The figure shows three views and two pictorial views of one solid part (mm, origin at its lowest corner). Answer the questions. Give positions to 0.01 mm unless a question says otherwise; leave off trailing zeros. Write each loop counter-clockwise with the first axis right and the second up, starting at its lowest first coordinate (ties: lowest second). Pieces come first, ordered by that corner, then holes. Notation, with made-up numbers: (23.5, -0.5) -> (32.5, -0.5) arc R35 ccw to (32.5, 34.5) -> close; hole circle Ø1 at (86.5, 7). An arc over 180 degrees is marked (long way). Use a Markdown table: item, result.
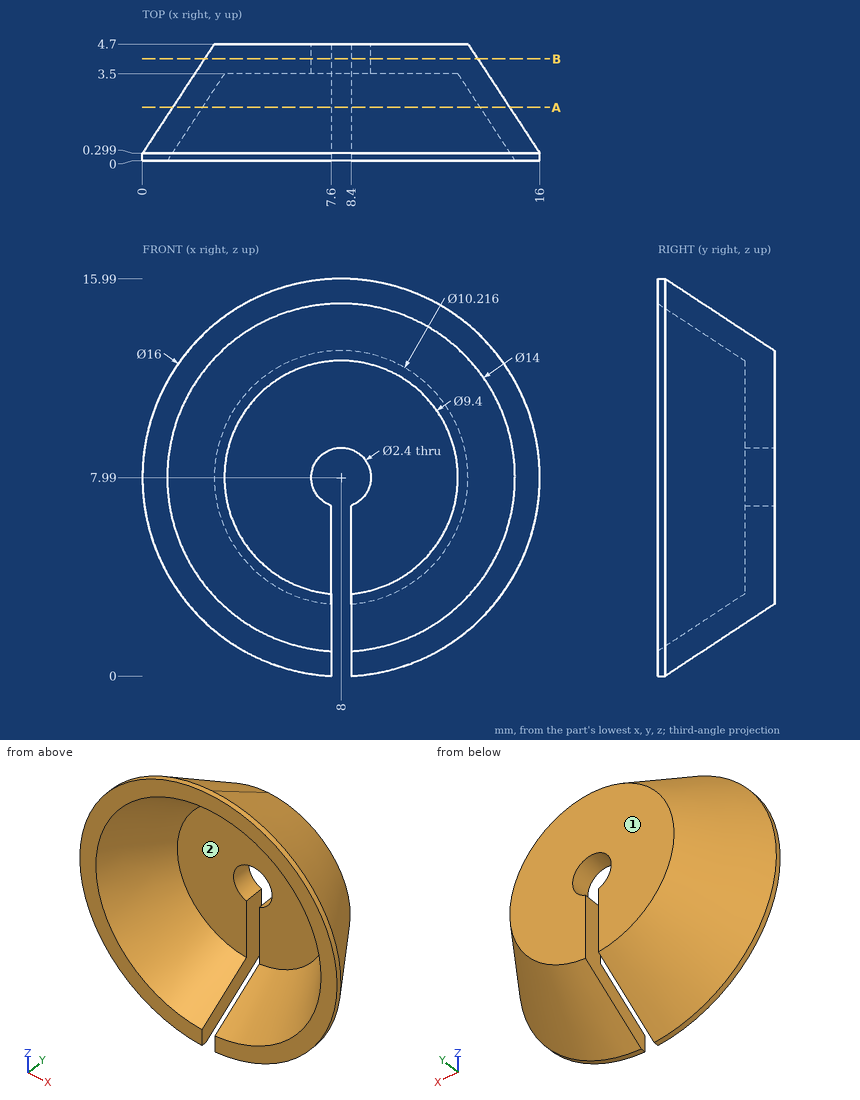
Item 1: Straight lines are drawn through the part: line 1 along Y through (x, z) = (10.5, 10.25); line 2 along Z through (x, y) = (6.25, 3.35); line 3 along Z through (x, y) = (9.75, 0.8). For each, find the intervals that lie inside material, in ascending order. Write a range as [from, to].
Return value:
| item | result |
|---|---|
| line 1 | [3.5, 4.7] |
| line 2 | [2.26, 3.52], [12.46, 13.72] |
| line 3 | [0.52, 1.76], [14.22, 15.46] |
Item 2: Each of these flat-tipped pins is pushed along its axis until it touches: P1, Ø7.5, axis at x = 6, z = 8, coming from the -Y side; P2, Ø3, axis at x = 8.5, z = 11, coming from the -Y side; P3, Ø2.5, axis at y = 2.5, z = 2, coming from the -X side (1 decimal); P4, Ø2, axis at x = 8, z = 7.99, coming from the +Y side. Where does it stop, or does it pass through?
Return value:
| item | result |
|---|---|
| P1 | y = 1.9 |
| P2 | y = 3.5 |
| P3 | x = 3 |
| P4 | through |
Item 3: For a pull along Z with two mould halves and no side action, classify the marked faces 1 and 2 as +Z half, -Z half, draft (parallel to the pull), parting line (faces both ways), or undercut.
Return value:
| item | result |
|---|---|
| face 1 | draft |
| face 2 | undercut |
Item 4: A cutting plane is placed at B-B (y = 4.1). Give the vertices of the cut face in (x, z), then the cut area to 3 significant figures.
Return value:
| item | result |
|---|---|
| outline | (7.6, 2.5) -> (7.6, 6.86) arc R1.2 cw (long way) to (8.4, 6.86) -> (8.4, 2.5) arc R5.5 ccw (long way) to start |
| area | 87.1 mm^2 |
Item 5: A cutting plane is placed at A-A (y = 2.15). Give the vertices of the cut face in (x, z).
Return value:
| item | result |
|---|---|
| outline | (7.6, 1.22) -> (7.6, 2.42) arc R5.59 cw (long way) to (8.4, 2.42) -> (8.4, 1.22) arc R6.78 ccw (long way) to start |
